```python
from build123d import *

# Parameters (mm, degrees)
SKETCH1_R           = 42
SKETCH1_R_2         = 33
BOSS_EXTRUDE1_DEPTH = 5
SKETCH9_R           = 1.5
CUT_EXTRUDE5_DEPTH  = 7
SKETCH10_R          = 2
CUT_EXTRUDE6_DEPTH  = 7


with BuildPart() as part:
    # Sketch1 → Boss-Extrude1 (new body)
    # profile 1 of 2: a face of its own
    with BuildSketch(Plane.XY):
        Circle(SKETCH1_R)
        Circle(SKETCH1_R_2, mode=Mode.SUBTRACT)
    # profile 2 of 2: a face of its own
    with BuildSketch(Plane.XY):
        with BuildLine():
            Line((-15, -80), (15, -80))
            Line((15, -80), (39.354283789, -14.67107179))
            ThreePointArc((39.354283789, -14.67107179), (0, -42), (-39.354283789, -14.67107179))
            Line((-39.354283789, -14.67107179), (-15, -80))
        make_face()
    extrude(amount=BOSS_EXTRUDE1_DEPTH)

    # Sketch9 → Cut-Extrude5 (cut)
    with BuildSketch(Plane.XY.offset(5)):
        with Locations((19, 32.908965344)):
            Circle(SKETCH9_R)
        with Locations((38, 0)):
            Circle(SKETCH9_R)
        with Locations((19, -32.908965344)):
            Circle(SKETCH9_R)
        with Locations((-19, -32.908965344)):
            Circle(SKETCH9_R)
        with Locations((-38, 0)):
            Circle(SKETCH9_R)
        with Locations((-19, 32.908965344)):
            Circle(SKETCH9_R)
    extrude(amount=-CUT_EXTRUDE5_DEPTH, mode=Mode.SUBTRACT)

    # Sketch10 → Cut-Extrude6 (cut)
    with BuildSketch(Plane.XY.offset(5)):
        with Locations((7.5, -60)):
            Circle(SKETCH10_R)
        with Locations((7.5, -70)):
            Circle(SKETCH10_R)
        with Locations((-7.5, -70)):
            Circle(SKETCH10_R)
        with Locations((-7.5, -60)):
            Circle(SKETCH10_R)
        with Locations((-7.5, -50)):
            Circle(SKETCH10_R)
        with Locations((7.5, -50)):
            Circle(SKETCH10_R)
    extrude(amount=-CUT_EXTRUDE6_DEPTH, mode=Mode.SUBTRACT)


solid = part.part
```
Geometry check sheet. Reference: the model listing, model coordinates, mm. Coordinates: 2 decimals unless noted, no trailing zeros. Order: outer loops, then holes, each group sorted by start corner. A loop starts at its lowest first (then second) coordinate and runs counter-clockwise, first axis right, second up.
Item 1: Depth check by flat-ended pin: pin 1 (1 mm diameter, centred on x = -33, z = 4, fed in from +Y); pin 2 (3 mm diameter, centred on x = -7.5, y = -50, fed in from +Z); pin 3 (1 mm diameter, centred on y = -21.5, z = 4, fed in from -X). Enter the tip coordinate at first touch or a pass-through.
Item 2: Scan lines: line 1 along Y through (x, z) = (-7.5, 3.8); line 2 along Y through (x, z) = (1, 2.4); line 3 along Y through (x, z) = (-8, 4.15). Record each from-to range of solid material in increasing order.
Item 3: Section check C-C (y = 9). Enter the section's corners in (x, z), plus the area to 3 significant figures.
Item 4: Section check A-A (y = -60). Enter the section's corners in (x, z).
Item 5: Mould release check, pull along X, two halves, no side actions. Record for faces 1 (the cylindrical face through (-7.934, -51.952, 2.535)), 2 (the flat face through (0, -80, 2)), 3 (the flat face through (27.007, -47.793, 2.465)): released by +X, released by -X, zero draft, split by the parting line, or undercut.
Item 6: Section check B-B (x = 11). Enter the section's corners in (y, z), plus the area to 3 significant figures.
Item 7: Section check D-D (x = -19). Enter the section's corners in (y, z), plus the area to 3 significant figures.
Check sheet entries:
1. pin 1: stops at y = 26.6
1. pin 2: passes through
1. pin 3: stops at x = -36.99
2. line 1: y = -80 to -72, -68 to -62, -58 to -52, -48 to -32.14, 32.14 to 41.32
2. line 2: y = -80 to -32.98, 32.98 to 41.99
2. line 3: y = -80 to -71.94, -68.06 to -61.94, -58.06 to -51.94, -48.06 to -32.02, 32.02 to 41.23
3. outline: (-41.02, 0) - (-31.75, 0) - (-31.75, 5) - (-41.02, 5) - close; (31.75, 0) - (41.02, 0) - (41.02, 5) - (31.75, 5) - close
3. area: 92.8 mm2
4. outline: (-22.46, 0) - (-9.5, 0) - (-9.5, 5) - (-22.46, 5) - close; (-5.5, 0) - (5.5, 0) - (5.5, 5) - (-5.5, 5) - close; (9.5, 0) - (22.46, 0) - (22.46, 5) - (9.5, 5) - close
5. face 1: undercut
5. face 2: zero draft
5. face 3: released by +X
6. outline: (-80, 0) - (-31.11, 0) - (-31.11, 5) - (-80, 5) - close; (31.11, 0) - (40.53, 0) - (40.53, 5) - (31.11, 5) - close
6. area: 292 mm2
7. outline: (-69.27, 0) - (-34.41, 0) - (-34.41, 5) - (-69.27, 5) - close; (-31.41, 0) - (-26.98, 0) - (-26.98, 5) - (-31.41, 5) - close; (26.98, 0) - (31.41, 0) - (31.41, 5) - (26.98, 5) - close; (34.41, 0) - (37.46, 0) - (37.46, 5) - (34.41, 5) - close
7. area: 234 mm2
